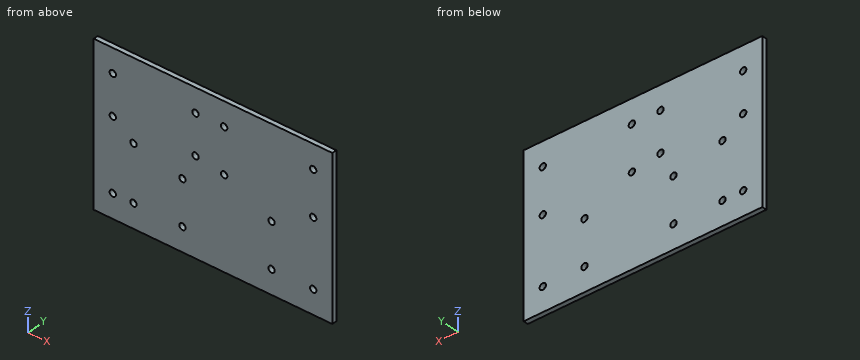
```python
from build123d import *

# Parameters (mm, degrees)
SKETCH1_W           = 150
SKETCH1_H           = 100
SKETCH1_R           = 2
BOSS_EXTRUDE1_DEPTH = 3
SKETCH2_R           = 2
CUT_EXTRUDE1_DEPTH  = 3


with BuildPart() as part:
    # Sketch1 → Boss-Extrude1 (new body)
    with BuildSketch(Plane(origin=(0, 0, 0), x_dir=(1, 0, 0), z_dir=(0, 1, 0))):
        with Locations((63, -37.502720101)):
            Rectangle(SKETCH1_W, SKETCH1_H)
        with Locations((0, -2.502720101)):
            Circle(SKETCH1_R, mode=Mode.SUBTRACT)
        with Locations((126, -2.502720101)):
            Circle(SKETCH1_R, mode=Mode.SUBTRACT)
        with Locations((0, -72.502720101)):
            Circle(SKETCH1_R, mode=Mode.SUBTRACT)
        with Locations((126, -72.502720101)):
            Circle(SKETCH1_R, mode=Mode.SUBTRACT)
    extrude(amount=BOSS_EXTRUDE1_DEPTH)

    # Sketch2 → Cut-Extrude1 (cut)
    with BuildSketch(Plane(origin=(0, 3, 0), x_dir=(1, 0, 0), z_dir=(0, 1, 0))):
        with Locations((13, -2.502720101)):
            Circle(SKETCH2_R)
        with Locations((13, -37.502720101)):
            Circle(SKETCH2_R)
        with Locations((0, -47.502720101)):
            Circle(SKETCH2_R)
        with Locations((0, -72.502720101)):
            Circle(SKETCH2_R)
        with Locations((52, -47.502720101)):
            Circle(SKETCH2_R)
        with Locations((52, -72.502720101)):
            Circle(SKETCH2_R)
        with Locations((43.800232524, -2.502720101)):
            Circle(SKETCH2_R)
        with Locations((43.800232524, -30.502720101)):
            Circle(SKETCH2_R)
        with Locations((99.800232524, -2.502720101)):
            Circle(SKETCH2_R)
        with Locations((99.800232524, -30.502720101)):
            Circle(SKETCH2_R)
        with Locations((70, -44.502720101)):
            Circle(SKETCH2_R)
        with Locations((70, -72.502720101)):
            Circle(SKETCH2_R)
        with Locations((126, -44.502720101)):
            Circle(SKETCH2_R)
    extrude(amount=-CUT_EXTRUDE1_DEPTH, mode=Mode.SUBTRACT)


solid = part.part
```
Input: part model. Units: mm. Frame: model coordinates. Coordinates: 2 decimals unless noted, no trailing zeros. Order: outer loops, then holes, each group sorted by start corner. A loop starts at its lowest first (then second) coordinate and runs counter-clockwise, first axis right, second up. Notation, with made-up numbers: (-27.75, 47) - (-2.75, 47) arc R29 ccw to (-2.75, 69) - close; hole circle Ø7 at (-15, 81.5). An arc over 180 degrees is marked (long way). Put each result on its own line as item: value.
1. Line query: line 1 along X through (y, z) = (0.5, 30.5); line 2 along Z through (x, y) = (52, 2); line 3 along Z through (x, y) = (70, 2.75). Output: solid intervals per line, ascending.
Report:
line 1: x = -12 to 41.8, 45.8 to 97.8, 101.8 to 138
line 2: z = -12.5 to 45.5, 49.5 to 70.5, 74.5 to 87.5
line 3: z = -12.5 to 42.5, 46.5 to 70.5, 74.5 to 87.5
2. Cut plane A-A on x = 126. Return the cut outline in (y, z), then the cut area to 3 significant figures.
Report:
outline: (0, -12.5) - (3, -12.5) - (3, 0.5) - (0, 0.5) - close; (0, 4.5) - (3, 4.5) - (3, 42.5) - (0, 42.5) - close; (0, 46.5) - (3, 46.5) - (3, 70.5) - (0, 70.5) - close; (0, 74.5) - (3, 74.5) - (3, 87.5) - (0, 87.5) - close
area: 264 mm2
3. Cut plane B-B on x = 52. Return the cut outline in (y, z), then the cut area to 3 significant figures.
Report:
outline: (0, -12.5) - (3, -12.5) - (3, 45.5) - (0, 45.5) - close; (0, 49.5) - (3, 49.5) - (3, 70.5) - (0, 70.5) - close; (0, 74.5) - (3, 74.5) - (3, 87.5) - (0, 87.5) - close
area: 276 mm2
